Geometry check sheet. Reference: the model listing, model coordinates, mm. Coordinates: 2 decimals unless noted, no trailing zeros. Order: outer loops, then holes, each group sorted by start corner. A loop starts at its lowest first (then second) coordinate and runs counter-clockwise, first axis right, second up. Notation, with made-up numbers: (75.25, 85) - (87.25, 85) arc R22 cw to (87.25, 105) - close; hole circle Ø7 at (-6, -15.5). An arc over 180 degrees is marked (long way). Return JSON: item names as keys, results as strings. Group by question number.
Item 1: Section check A-A on y = 0.6. Enter the section's corners in (x, z) (3 decimals), then the cut area to 3 significant figures.
Item 2: Gauge pin test, flat end, axial feed: pin 1 (0.8 mm diameter, centred on x = -53, y = 1, fed in from +Z). Record the tip position at first contact, or that the pin passes through.
Item 3: Section check B-B on x = -49.5. Enter the section's corners in (y, z), then the cut area to 3 significant figures.
Item 4: Scan lines: probe 1 along Z at (x, y) = (15.5, 0.3); probe 2 along X at (y, z) = (1.2, 26). Record each from-to range of solid material in increasing order.
from build123d import *

# Parameters (mm, degrees)
BOSS_EXTRUDE1_DEPTH       = 1.6256
F_4_CLEARANCE_HOLE1_D     = 3.2639
F_4_CLEARANCE_HOLE1_DEPTH = 56.388
F_4_CLEARANCE_HOLE1_TIP   = 0.980574487


with BuildPart() as part:
    # Sketch1 → Boss-Extrude1 (new body)
    with BuildSketch(Plane(origin=(0, 0, 0), x_dir=(1, 0, 0), z_dir=(0, 1, 0))):
        Polygon((60.96, 31.75), (19.558, 31.75), (-17.272, 31.75), (-60.96, 31.75), (-60.96, -23.7998), (-35.09199383, -23.7998), (-35.09199383, -31.75), (6.64020617, -31.75), (6.64020617, -23.7998), (60.96, -23.7998), align=None)
    extrude(amount=BOSS_EXTRUDE1_DEPTH)

    # #4 Clearance Hole1
    with Locations(Plane(origin=(-46.701329526, 0, 29.554902493), x_dir=(-1, 0, 0), z_dir=(0, -1, 0))):
        with Locations((-102.911529526, 9.869902493), (-102.911529526, 56.859902493), (9.686670474, 56.859902493), (9.686670474, 9.869902493)):
            Hole(F_4_CLEARANCE_HOLE1_D / 2, depth=F_4_CLEARANCE_HOLE1_DEPTH)
            with Locations((0, 0, -(F_4_CLEARANCE_HOLE1_DEPTH + F_4_CLEARANCE_HOLE1_TIP / 2))):  # 118° drill point
                Cone(0, F_4_CLEARANCE_HOLE1_D / 2, F_4_CLEARANCE_HOLE1_TIP, mode=Mode.SUBTRACT)


solid = part.part
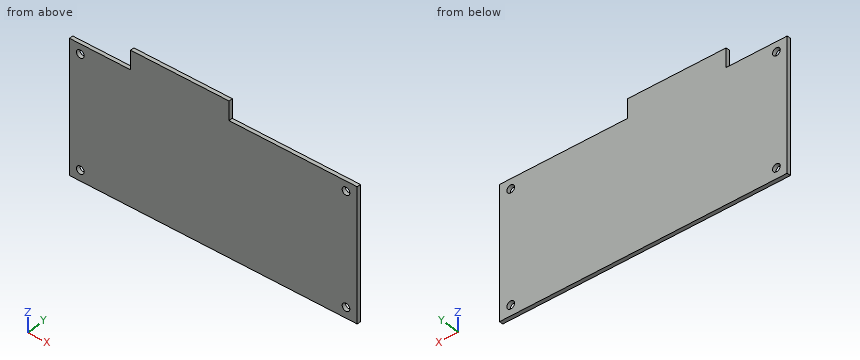
Computed:
{
 "1": {"outline": "(-60.96, -31.75) - (60.96, -31.75) - (60.96, 23.8) - (6.64, 23.8) - (6.64, 31.75) - (-35.092, 31.75) - (-35.092, 23.8) - (-60.96, 23.8) - close; hole circle Ø3.264 at (-56.388, -27.305); hole circle Ø3.264 at (-56.388, 19.685); hole circle Ø3.264 at (56.21, -27.305); hole circle Ø3.264 at (56.21, 19.685)", "area": "7,070 mm²"},
 "2": {"pin 1": "stops at z = 23.8"},
 "3": {"outline": "(0, -31.75) - (1.63, -31.75) - (1.63, 23.8) - (0, 23.8) - close", "area": "90.3 mm²"},
 "4": {"probe 1": "z = -31.75 to 23.8", "probe 2": "x = -35.09 to 6.64"}
}
